```python
from build123d import *

# Parameters (mm, degrees)
SKETCH1_W            = 75
SKETCH1_H            = 50
BOSS_EXTRUDE1_DEPTH  = 15
CHAMFER1_SIZE        = 2
SKETCH2_W            = 22
SKETCH2_H            = 9
BOSS_EXTRUDE2_DEPTH  = 20
SKETCH3_R            = 11
BOSS_EXTRUDE3_DEPTH  = 21
SKETCH4_R            = 4
CUT_EXTRUDE2_DEPTH   = 94.968079687
SKETCH4_4_R          = 7.5
SKETCH4_4_R_2        = 4
CUT_EXTRUDE3_DEPTH   = 6
FILLET1_R            = 3
LPATTERN2_COUNT      = 2
LPATTERN2_PITCH      = 52
LPATTERN2_COUNT_DIR2 = 2
LPATTERN2_PITCH_DIR2 = 25


with BuildPart() as part:
    # Sketch1 → Boss-Extrude1 (new body)
    with BuildSketch(Plane(origin=(0, 0, 0), x_dir=(1, 0, 0), z_dir=(0, 1, 0))):
        with Locations((37.5, 25)):
            Rectangle(SKETCH1_W, SKETCH1_H)
    extrude(amount=BOSS_EXTRUDE1_DEPTH)

    # Chamfer1
    chamfer1_edges = [part.edges().sort_by_distance(p)[0] for p in [
        (37.5, 15, 0),
        (0, 15, -25),
        (37.5, 15, -50),
        (75, 15, -25),
    ]]
    chamfer(chamfer1_edges, length=CHAMFER1_SIZE)

    # Sketch2 → Boss-Extrude2 (add)
    with BuildSketch(Plane(origin=(0, 15, 0), x_dir=(1, 0, 0), z_dir=(0, 1, 0))):
        with Locations((37.5, 33.5)):
            Rectangle(SKETCH2_W, SKETCH2_H)
    extrude(amount=BOSS_EXTRUDE2_DEPTH)

    # Sketch3 → Boss-Extrude3 (add)
    with BuildSketch(Plane(origin=(0, 0, -38), x_dir=(-1, 0, 0), z_dir=(0, 0, -1))):
        with Locations((-37.5, 35)):
            Circle(SKETCH3_R)
    extrude(amount=-BOSS_EXTRUDE3_DEPTH)

    # Sketch4 → Cut-Extrude2 (cut, through all)
    with BuildSketch(Plane.XY.offset(-17)):
        with Locations((37.5, 35)):
            Circle(SKETCH4_R)
    extrude(amount=-CUT_EXTRUDE2_DEPTH, mode=Mode.SUBTRACT)

    # Sketch4<4> → Cut-Extrude3 (cut)
    with BuildSketch(Plane.XY.offset(-17)):
        with Locations((37.5, 35)):
            Circle(SKETCH4_4_R)
        with Locations((37.5, 35)):
            Circle(SKETCH4_4_R_2, mode=Mode.SUBTRACT)
    extrude(amount=-CUT_EXTRUDE3_DEPTH, mode=Mode.SUBTRACT)

    # Fillet1
    fillet1_edges = [part.edges().sort_by_distance(p)[0] for p in [
        (37.5, 15, -29),
        (26.5, 15, -33.5),
        (37.5, 15, -38),
        (48.5, 15, -33.5),
    ]]
    fillet(fillet1_edges, radius=FILLET1_R)

    # Sketch10 → CBORE for M6 Hex Head Bolt2 (revolve, cut)
    with BuildSketch(Plane(origin=(63.5, 15, -37), x_dir=(0, 0, 1), z_dir=(1, 0, 0))):
        Polygon((0, 0), (0, 15), (3.3, 15), (3.3, 4.405), (3.325, 4.38), (7.275, 4.38), (7.275, 0.025), (7.3, 0), align=None)
    cbore_for_m6_hex_head_bolt2 = revolve(axis=Axis((63.5, 21.35, -37), (0, -1, 0)), mode=Mode.SUBTRACT)

    # LPattern2: CBORE for M6 Hex Head Bolt2 2 × 2
    with Locations(*[(-i * LPATTERN2_PITCH, 0, j * LPATTERN2_PITCH_DIR2) for i in range(LPATTERN2_COUNT) for j in range(LPATTERN2_COUNT_DIR2) if (i, j) != (0, 0)]):
        add(cbore_for_m6_hex_head_bolt2, mode=Mode.SUBTRACT)


solid = part.part
```
Build history of the part. All positions in model axes, mm. A direction names the side the tool comes from. Round coordinates to 2 decimals unless told otherwise and drop trailing zeros. Write each loop counter-clockwise with the first axis right and the second up, starting at its lowest first coordinate (ties: lowest second). Pieces come first, ordered by that corner, then holes. Notation, with made-up numbers: (86, 65.5) - (113, 65.5) arc R10 cw to (113, 72.5) - close; hole circle Ø10 at (22.25, -23). An arc over 180 degrees is marked (long way). Write each question's results on one line, items separated by ' | '. Start each with the question number.
Item 1: Which spindle directions (+Z, -Z, +X, -X, +Y, -Y) get a long thin tool onto all of the face, cutting with end or side? Do faces 4 (the face through (30, 33, -17)), 5 (the face through (11.18, 12.828, -19.268)), 6 (the face through (60.23, 5.37, -12.43)), 7 (the face through (48.5, 26, -33)), 8 (the face through (35.87, 27.68, -19.96)). Say none if no direction does.
Item 2: Wall check: L1, parallel to X at y = 13, z = -37 (3 decimals); L2, parallel to Y at x = 37, z = -18; L3, parallel to Z at x = 63, y = 13. Give the ranges that are in metal, low to high. Write a range as [from, to].
Item 3: Drop flat-ended pins along their axis: P1, Ø16.5, axis at x = 39.5, y = 34, coming from the +Z side; P2, Ø2, axis at y = 5, z = -13, coming from the -X side; P3, Ø3, axis at x = 64.5, z = -31.5, coming from the +Y side; P4, Ø7, axis at y = 29, z = -35, coming from the -X side. Give the stop position or say it passes through.
Item 4: Mould opens along Z. For faces 1 (the face through (41, 32, -23)), 2 (the face through (37, 29, -38)), 3 (the face through (67, 10.62, -14)) say: pulls with the +Z half, pulls with the -Z half, needs draft (parallel to the pull), parting line crosses it, or undercut.
Item 5: Saw through at B-B (z = -12). State how many separate pieces and enclosed holes the cut face has, and give its area (3 significant figures).
Item 6: Saw through at A-A (x = 37.5). Write the cut outline in (y, z).
Results are:
1) face 4: +Z, +X, -X, +Y | face 5: +Y | face 6: +Y, -Y | face 7: +Z, -Z, +X, +Y | face 8: +Z
2) L1: x = [0, 4.225], [18.775, 56.225], [70.775, 75] | L2: y = [0, 15], [24.01, 27.52], [42.48, 45.99] | L3: z = [-50, -44.26], [-29.74, -19.26], [-4.74, 0]
3) P1: stops at z = -17 | P2: stops at x = 0 | P3: stops at y = 10.62 | P4: stops at x = 26.5
4) face 1: pulls with the +Z half | face 2: pulls with the -Z half | face 3: undercut
5) separate pieces: 3 | enclosed holes: 0 | area: 853 mm²
6) outline: (0, -50) - (13, -50) - (15, -48) - (15, -41) arc R3 cw to (18, -38) - (31, -38) - (31, -23) - (27.5, -23) - (27.5, -17) - (24, -17) - (24, -29) - (18, -29) arc R3 cw to (15, -26) - (15, -2) - (13, 0) - (0, 0) - close; (39, -38) - (46, -38) - (46, -17) - (42.5, -17) - (42.5, -23) - (39, -23) - close
